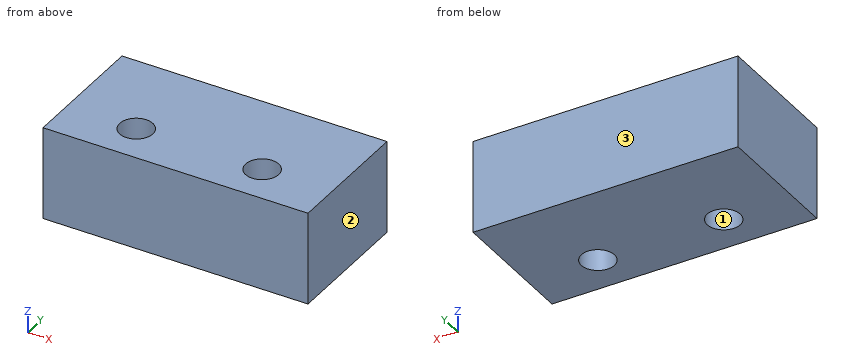
from build123d import *

# Parameters (mm, degrees)
CROQUIS1_W              = 20
CROQUIS1_H              = 7
SALIENTE_EXTRUIR1_DEPTH = 10
TALADRO1_D              = 2.5


with BuildPart() as part:
    # Croquis1 → Saliente-Extruir1 (new body)
    with BuildSketch(Plane(origin=(0, 0, 0), x_dir=(1, 0, 0), z_dir=(0, 1, 0))):
        Rectangle(CROQUIS1_W, CROQUIS1_H)
    extrude(amount=SALIENTE_EXTRUIR1_DEPTH)

    # Taladro1 (through all)
    with Locations(Plane.XY.offset(3.5)):
        with Locations((-4.75, 3), (4.75, 3)):
            Hole(TALADRO1_D / 2)


solid = part.part
Could you check a few things on this model? Use its own coordinates, in mm. Face numbers are marked on the shaded views. Give positions to 0.01 mm unless a question says otherwise; leave off trailing zeros. Order: outer loops, then holes, each group sorted by start corner. A loop starts at its lowest first (then second) coordinate and runs counter-clockwise, first axis right, second up.
Item 1: If we section it at C-C, the plane z = -0.5: Write out the boundary of the cut face in (x, y).
Item 2: If we mould it in two halves opening along X, with no side actions, what happens to the marked faces 1, 2 and 3? For each: pulls with the +X half, pulls with the -X half, needs draft (parallel to the pull), parting line crosses it, or undercut.
Item 3: If we section it at A-A, the plane x = -5.75: Write out the boundary of the cut face in (y, z), plus the area to 3 significant figures.
Item 4: If we section it at B-B, the plane y = 3: Write out the boundary of the cut face in (x, z), plus the area to 3 significant figures.
Item 5: I need wall thicknesses on line 1 (Y direction, x = -4.75, z = 0.25); line 2 (X direction, y = 4, z = -2.5); line 3 (X direction, y = 2.5, z = 2.25). Which ranges of each line are inside material? Lowest first, please.
Item 6: If we section it at D-D, the plane x = 4.75: Write out the boundary of the cut face in (y, z), plus the area to 3 significant figures.
Values:
1. outline: (-10, 0) - (10, 0) - (10, 10) - (-10, 10) - close; hole circle Ø2.5 at (-4.75, 3); hole circle Ø2.5 at (4.75, 3)
2. face 1: undercut
2. face 2: pulls with the +X half
2. face 3: needs draft
3. outline: (0, -3.5) - (2.25, -3.5) - (2.25, 3.5) - (0, 3.5) - close; (3.75, -3.5) - (10, -3.5) - (10, 3.5) - (3.75, 3.5) - close
3. area: 59.5 mm2
4. outline: (-10, -3.5) - (-6, -3.5) - (-6, 3.5) - (-10, 3.5) - close; (-3.5, -3.5) - (3.5, -3.5) - (3.5, 3.5) - (-3.5, 3.5) - close; (6, -3.5) - (10, -3.5) - (10, 3.5) - (6, 3.5) - close
4. area: 105 mm2
5. line 1: y = 0 to 1.75, 4.25 to 10
5. line 2: x = -10 to -5.5, -4 to 4, 5.5 to 10
5. line 3: x = -10 to -5.9, -3.6 to 3.6, 5.9 to 10
6. outline: (0, -3.5) - (1.75, -3.5) - (1.75, 3.5) - (0, 3.5) - close; (4.25, -3.5) - (10, -3.5) - (10, 3.5) - (4.25, 3.5) - close
6. area: 52.5 mm2
